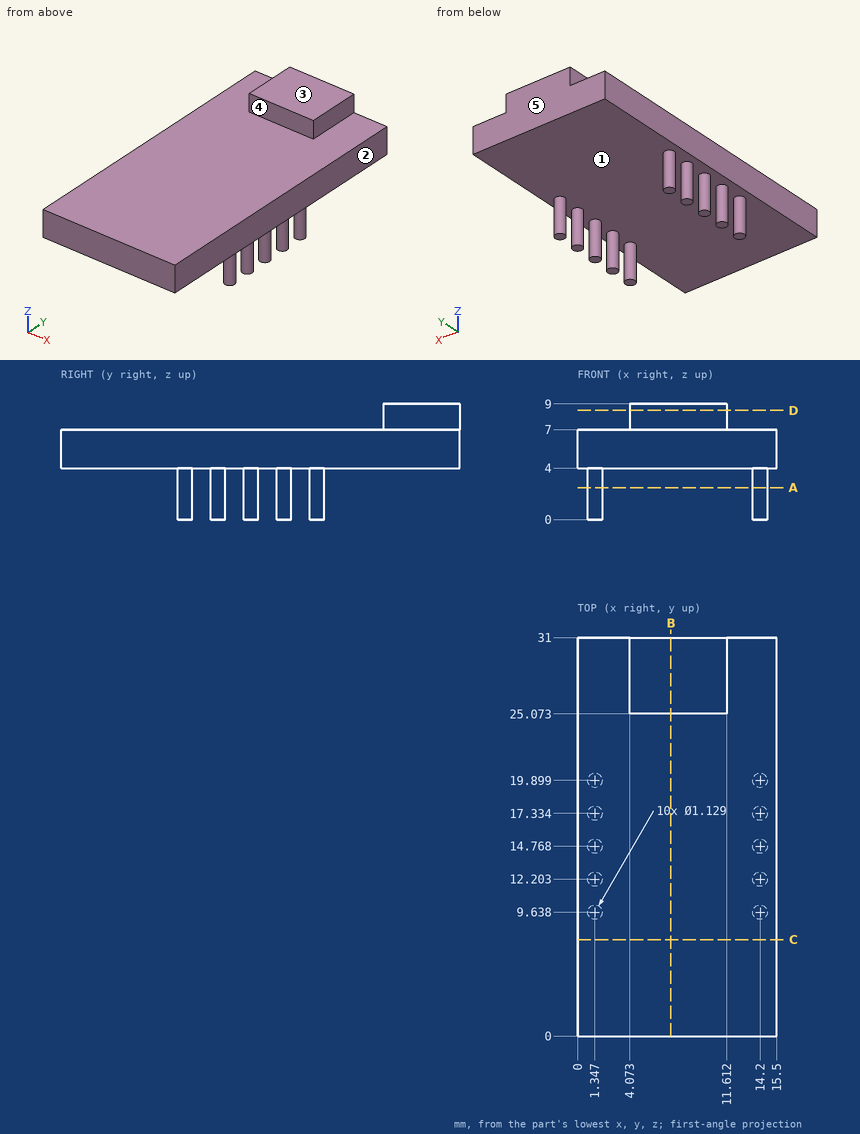
Geometry: see drawing. Coordinates: mm, zero at the bounding-box minimum. A direction names the side the tool comes from. Coordinates: 2 decimals unless noted, no trailing zeros. Loops run counter-clockwise (first coordinate to the right, second up) from the corner with the lowest first, then second, coordinate; pieces in that order, holes last.
Q1. Set-up query: the marked faces 4 and 5. Return all of +Z, -Z, +X, -X, +Y, -Y with unobstructed straight access to the full face (end or side cutting, diameter ignored); none if empty.
Q2. Cut plane B-B (x = 7.25). Output: boundary loops of the cut face in (y, z), then the cut area to 3 significant figures.
Q3. Cut plane C-C (y = 7.5). Output: boundary loops of the cut face in (x, z).
Q4. Cut plane D-D (z = 8.5). Output: boundary loops of the cut face in (x, y), then the cut area to 3 significant figures.
Q5. Contact query for flat-ended pins moving along their axis: pin 1 (5 mm diameter, centred on y = 3.5, z = 3, fed in from -X); pin 2 (1 mm diameter, centred on y = 28.5, z = 8, fed in from +X); pin 3 (2 mm diameter, centred on x = 3.5, y = 3.5, fed in from -Z); pin 4 (1.5 mm diameter, centred on y = 5, z = 2, fed in from -X). Output: stop coordinate, or through.
Q6. Draft query along Z for the marked faces 1, 2 and 3. Return one class per face: +Z half, -Z half, draft (parallel to the pull), parting line (faces both ways), or undercut.
Q7. Material intervals for line 1 (Z direction, x = 10.25, y = 12); line 2 (X direction, y = 26.5, z = 7.75); line 3 (Z direction, x = 5, y = 26), sorted ascending.
Q8. Cut plane A-A (z = 2.5). Give the number of separate pieces and of enclosed holes in the cut face, then the cut area to 3 significant figures.
Working result:
1. face 4: +Z, +X, -X, -Y
1. face 5: +Z, -Z, +X, -X, +Y
2. outline: (0, 4) - (31, 4) - (31, 9) - (25.07, 9) - (25.07, 7) - (0, 7) - close
2. area: 105 mm2
3. outline: (0, 4) - (15.5, 4) - (15.5, 7) - (0, 7) - close
4. outline: (4.07, 25.07) - (11.61, 25.07) - (11.61, 31) - (4.07, 31) - close
4. area: 44.7 mm2
5. pin 1: stops at x = 0
5. pin 2: stops at x = 11.61
5. pin 3: stops at z = 4
5. pin 4: passes through
6. face 1: -Z half
6. face 2: draft
6. face 3: +Z half
7. line 1: z = 4 to 7
7. line 2: x = 4.07 to 11.61
7. line 3: z = 4 to 9
8. separate pieces: 10
8. enclosed holes: 0
8. area: 10.0 mm2
